```python
from build123d import *

# Parameters (mm, degrees)
F0_R     = 12.7
F0_R_2   = 44.45
F1_DEPTH = 6.35


# Not quite as in the source:
# - a length typed as a fraction of an inch, garbled in the dataset ("3 / 203.2 mm" for 3/8 in), is restored


with BuildPart() as f1:
    # F0 (on Top) → F1 (new body)
    with BuildSketch(Plane.XY):
        with BuildLine():
            ThreePointArc((-74.5464027897, -31.7069095982), (-59.4196204119, -34.5232781397), (-46.6403597532, -43.0931074194))
            ThreePointArc((-46.6403597532, -43.0931074194), (-46.1303112619, -43.6221670242), (-45.6305618227, -44.160965713))
            ThreePointArc((-45.6305618227, -44.160965713), (0, -63.500701295), (45.6305618227, -44.160965713))
            ThreePointArc((45.6305618227, -44.160965713), (46.1303112619, -43.6221670242), (46.6403597532, -43.0931074194))
            ThreePointArc((46.6403597532, -43.0931074194), (59.4196204119, -34.5232781397), (74.5464027897, -31.7069095982))
            ThreePointArc((74.5464027897, -31.7069095982), (75.115235957, -31.7221094671), (75.6837786723, -31.745803117))
            ThreePointArc((75.6837786723, -31.745803117), (107.95, 0), (75.6837786723, 31.745803117))
            ThreePointArc((75.6837786723, 31.745803117), (75.115235957, 31.7221094671), (74.5464027897, 31.7069095982))
            ThreePointArc((74.5464027897, 31.7069095982), (59.4196204119, 34.5232781397), (46.6403597532, 43.0931074194))
            ThreePointArc((46.6403597532, 43.0931074194), (46.1303112619, 43.6221670242), (45.6305618227, 44.160965713))
            ThreePointArc((45.6305618227, 44.160965713), (0, 63.500701295), (-45.6305618227, 44.160965713))
            ThreePointArc((-45.6305618227, 44.160965713), (-46.1303112619, 43.6221670242), (-46.6403597532, 43.0931074194))
            ThreePointArc((-46.6403597532, 43.0931074194), (-59.4196204119, 34.5232781397), (-74.5464027897, 31.7069095982))
            ThreePointArc((-74.5464027897, 31.7069095982), (-75.115235957, 31.7221094671), (-75.6837786723, 31.745803117))
            ThreePointArc((-75.6837786723, 31.745803117), (-107.95, 0), (-75.6837786723, -31.745803117))
            ThreePointArc((-75.6837786723, -31.745803117), (-75.115235957, -31.7221094671), (-74.5464027897, -31.7069095982))
        make_face()
        with Locations((-76.2, 0)):
            Circle(F0_R, mode=Mode.SUBTRACT)
        Circle(F0_R_2, mode=Mode.SUBTRACT)
        with BuildLine():
            ThreePointArc((63.5005844158, 0.1218352114), (76.2609183065, 12.6998538952), (88.9, 0))
            ThreePointArc((88.9, 0), (76.2609183065, -12.6998538952), (63.5005844158, -0.1218352114))
            ThreePointArc((63.5005844158, -0.1218352114), (63.5, 0), (63.5005844158, 0.1218352114))
        make_face(mode=Mode.SUBTRACT)
    extrude(amount=F1_DEPTH)


solid = f1.part
```
Check sheet for the modelled part. Datum: model origin and axes. Units: mm. Give positions to 0.01 mm unless a question says otherwise; leave off trailing zeros. Order: outer loops, then holes, each group sorted by start corner. A loop starts at its lowest first (then second) coordinate and runs counter-clockwise, first axis right, second up. Notation, with made-up numbers: (15.25, 23) -> (26.25, 23) arc R19 cw to (26.25, 57) -> close; hole circle Ø5 at (25, -18.75). An arc over 180 degrees is marked (long way). Use CSV: the item, a comma, the result in double quotes. Start each with the question number.
1) Material ranges on line 1 (Y direction, x = 76.2, z = 3.75); line 2 (Y direction, x = -24, z = 2.75); line 3 (X direction, y = 39, z = 1.25), recorded low to high. Write a range as from..to.
2) Sectioned sample at A-A, the plane x = 0. Record the boundary of the cut face in (y, z).
3) Mould release check, pull along Y, two halves, no side actions. Record for faces 1 (the face through (42.397, 13.352, 3.131)), 2 (the face through (46, 1, 6.35)), 3 (the face through (-0.713, -63.497, 3.131)): released by +Y, released by -Y, zero draft, split by the parting line, or undercut.
4) Sectioned sample at D-D, the plane x = -59. Record the boundary of the cut face in (y, z), plus the area to 3 significant figures.
5) Go/stop test with flat-tipped pins: P1, Ø2, axis at x = 79, z = 2.5, coming from the -Y side; P2, Ø1.5, axis at y = -6, z = 2, coming from the +X side; P3, Ø2, axis at y = -7.5, z = 5.5, coming from the +X side. Record where each tip stops, or that it passes through.
6) Sectioned sample at C-C, the plane y = -41. Record the boundary of the cut face in (x, z).
Recorded:
1,line 1,"-31.75..-12.7, 12.7..31.75"
1,line 2,"-58.79..-37.41, 37.41..58.79"
1,line 3,"-51.39..-21.33, 21.33..51.39"
2,outline,"(-63.5, 0) -> (-44.45, 0) -> (-44.45, 6.35) -> (-63.5, 6.35) -> close; (44.45, 0) -> (63.5, 0) -> (63.5, 6.35) -> (44.45, 6.35) -> close"
3,face 1,"undercut"
3,face 2,"zero draft"
3,face 3,"released by -Y"
4,outline,"(-34.7, 0) -> (34.7, 0) -> (34.7, 6.35) -> (-34.7, 6.35) -> close"
4,area,"441 mm2"
5,P1,"y = -31.7"
5,P2,"x = 107.51"
5,P3,"x = 107.28"
6,outline,"(-48.87, 0) -> (-17.17, 0) -> (-17.17, 6.35) -> (-48.87, 6.35) -> close; (17.17, 0) -> (48.87, 0) -> (48.87, 6.35) -> (17.17, 6.35) -> close"
